Source: CAD feature listing. Evaluate the final solid. Frame: model axes, mm. Round coordinates to 2 decimals unless told otherwise and drop trailing zeros. Loops run counter-clockwise (first coordinate to the right, second up) from the corner with the lowest first, then second, coordinate; pieces in that order, holes last. Notation, with made-up numbers: M -36.5,-21 L 0.5,-21 A9 cw 0.5,-5 Z; hole C -15,31 d1. An arc over 180 degrees is marked long. Answer as a JSON object with one key per item and string values.
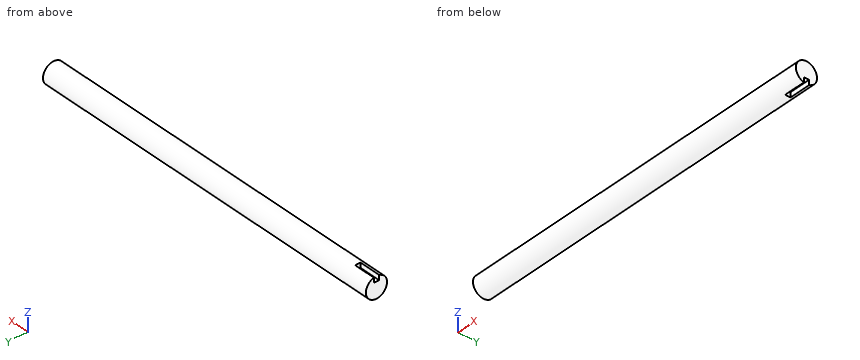
from build123d import *

# Parameters (mm, degrees)
SKETCH1_R           = 10
BOSS_EXTRUDE1_DEPTH = 350
SKETCH2_W           = 10
SKETCH2_H           = 5
CUT_EXTRUDE1_DEPTH  = 20
SKETCH3_W           = 10
SKETCH3_H           = 5
CUT_EXTRUDE2_DEPTH  = 20


with BuildPart() as part:
    # Sketch1 → Boss-Extrude1 (new body)
    with BuildSketch(Plane(origin=(0, 0, 0), x_dir=(0, 0, -1), z_dir=(1, 0, 0))):
        Circle(SKETCH1_R)
    extrude(amount=BOSS_EXTRUDE1_DEPTH)

    # Sketch2 → Cut-Extrude1 (cut)
    with BuildSketch(Plane.ZY):
        with Locations((10, 0)):
            Rectangle(SKETCH2_W, SKETCH2_H)
    extrude(amount=-CUT_EXTRUDE1_DEPTH, mode=Mode.SUBTRACT)

    # Sketch3 → Cut-Extrude2 (cut)
    with BuildSketch(Plane(origin=(350, 0, 0), x_dir=(0, 0, -1), z_dir=(1, 0, 0))):
        with Locations((10, 0)):
            Rectangle(SKETCH3_W, SKETCH3_H)
    extrude(amount=-CUT_EXTRUDE2_DEPTH, mode=Mode.SUBTRACT)


solid = part.part
Item 1: Line query: probe 1 along Z at (x, y) = (332.5, 0.5); probe 2 along Z at (x, y) = (52, -2.75); probe 3 along X at (y, z) = (1, -5.25). Output: solid intervals per line, ascending. Write a range as from..to.
Answer sheet:
{"probe 1": "z = -5..9.99", "probe 2": "z = -9.61..9.61", "probe 3": "x = 0..330"}
Item 2: Section A-A on x = 294. Return the cut outline in (y, z).
Answer sheet:
{"outline": "C 0,0 d20"}
Item 3: Contact query for flat-ended pins moving along their axis: pin 1 Ø1.4 at (x, z) = (339.5, -7) entering from -Y; pin 2 Ø6 at (x, y) = (114, 6.5) entering from -Z; pin 3 Ø1.5 at (y, z) = (-1, 8) entering from -X. Output: stop coordinate, or through.
Answer sheet:
{"pin 1": "stops at y = -7.77", "pin 2": "stops at z = -9.37", "pin 3": "stops at x = 20"}
Item 4: Section B-B on y = -6.25. Return the cut outline in (x, z), then the cut area to 3 significant figures.
Answer sheet:
{"outline": "M 0,-7.81 L 350,-7.81 L 350,7.81 L 0,7.81 Z", "area": "5,460 mm²"}
